Here's how the part is built. I have some questions about the finished solid (model axes, mm). Coordinates: 2 decimals unless noted, no trailing zeros. Loops run counter-clockwise (first coordinate to the right, second up) from the corner with the lowest first, then second, coordinate; pieces in that order, holes last. Notation, with made-up numbers: (36.25, 1) -> (47.25, 1) arc R27 cw to (47.25, 39) -> close; hole circle Ø11 at (-7.75, 75). An arc over 180 degrees is marked (long way). Answer as a JSON object with one key per item and string values. Group by question number.
1) I'm going to push a flat-ended pin straight in: pin 1 (1.9 mm diameter, centred on x = -181.44, z = -97.5, fed in from +Y). Where does the tip first touch, or does it pass through?
2) I need wall thicknesses on probe 1 along X at (y, z) = (1.35, -97.5); probe 2 along X at (y, z) = (1.5, -86); probe 3 along X at (y, z) = (1.6, -48). Which ranges of each line are inside material? Lowest first, please. Write a range as [from, to].
3) I want a section at A-A (z = -86). Write out the boundary of the cut face in (x, y), then the cut area to 3 significant figures.
4) I want a section at B-B (y = 0.65). Count the separate pieces of the cut face and the enclosed holes in it, then the cut area to 3 significant figures.
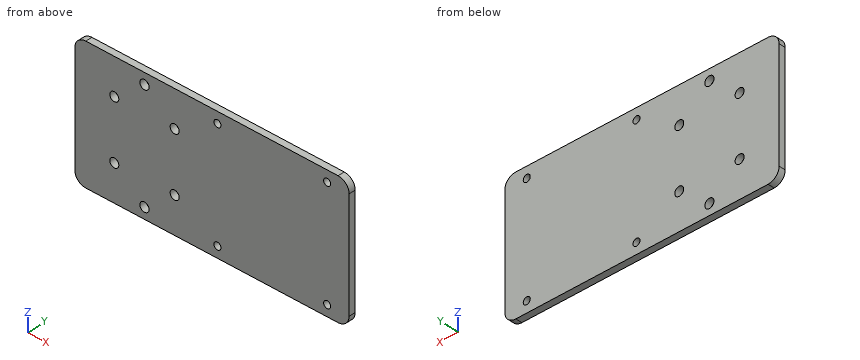
```python
from build123d import *

# Parameters (mm, degrees)
SKETCH_1_W          = 125
SKETCH_1_H          = 60
EXTRUDE_1_DEPTH     = 3
SKETCH_2_R          = 2.05
SKETCH_2_R_2        = 2.1
CUT_EXTRUDE_1_DEPTH = 267.924326413
SKETCH_3_R          = 1.6
CUT_EXTRUDE_2_DEPTH = 267.924326413
FILLET_1_R          = 5


with BuildPart() as part:
    # 草图1 → 凸台-拉伸1 (new body)
    with BuildSketch(Plane(origin=(0, 0, 0), x_dir=(1, 0, 0), z_dir=(0, 1, 0))):
        with Locations((-183.941364286, 72.5)):
            Rectangle(SKETCH_1_W, SKETCH_1_H)
    extrude(amount=EXTRUDE_1_DEPTH)

    # 草图2 → 切除-拉伸1 (cut, through all)
    with BuildSketch(Plane(origin=(0, 3, 0), x_dir=(1, 0, 0), z_dir=(0, 1, 0))):
        with Locations(Location((-228.441364286, 86, 0), (0, 0, 270))):
            Circle(SKETCH_2_R)
        with Locations(Location((-228.441364286, 59, 0), (0, 0, 270))):
            Circle(SKETCH_2_R)
        with Locations(Location((-200.941364286, 86, 0), (0, 0, 270))):
            Circle(SKETCH_2_R)
        with Locations(Location((-200.941364286, 59, 0), (0, 0, 90))):
            Circle(SKETCH_2_R)
        with Locations(Location((-214.691364286, 97.5, 0), (0, 0, 270))):
            Circle(SKETCH_2_R_2)
        with Locations(Location((-214.691364286, 47.5, 0), (0, 0, 90))):
            Circle(SKETCH_2_R_2)
    extrude(amount=-CUT_EXTRUDE_1_DEPTH, mode=Mode.SUBTRACT)

    # 草图3 → 切除-拉伸2 (cut, through all)
    with BuildSketch(Plane(origin=(0, 3, 0), x_dir=(1, 0, 0), z_dir=(0, 1, 0))):
        with Locations(Location((-181.441364286, 97.5, 0), (0, 0, 270))):
            Circle(SKETCH_3_R)
        with Locations(Location((-131.441364286, 97.5, 0), (0, 0, 270))):
            Circle(SKETCH_3_R)
        with Locations(Location((-131.441364286, 47.5, 0), (0, 0, 90))):
            Circle(SKETCH_3_R)
        with Locations(Location((-181.441364286, 47.5, 0), (0, 0, 90))):
            Circle(SKETCH_3_R)
    extrude(amount=-CUT_EXTRUDE_2_DEPTH, mode=Mode.SUBTRACT)

    # 圆角1
    fillet_1_edges = [part.edges().sort_by_distance(p)[0] for p in [
        (-121.441364286, 1.5, -42.5),
        (-246.441364286, 1.5, -42.5),
        (-246.441364286, 1.5, -102.5),
        (-121.441364286, 1.5, -102.5),
    ]]
    fillet(fillet_1_edges, radius=FILLET_1_R)


solid = part.part
```
Determined:
{
 "1": {"pin 1": "through"},
 "2": {"probe 1": "[-246.44, -216.79], [-212.59, -183.04], [-179.84, -133.04], [-129.84, -121.44]", "probe 2": "[-246.44, -230.49], [-226.39, -202.99], [-198.89, -121.44]", "probe 3": "[-246.44, -216.73], [-212.65, -182.96], [-179.92, -132.96], [-129.92, -121.44]"},
 "3": {"outline": "(-246.44, 0) -> (-230.49, 0) -> (-230.49, 3) -> (-246.44, 3) -> close; (-226.39, 0) -> (-202.99, 0) -> (-202.99, 3) -> (-226.39, 3) -> close; (-198.89, 0) -> (-121.44, 0) -> (-121.44, 3) -> (-198.89, 3) -> close", "area": "350 mm^2"},
 "4": {"separate pieces": "1", "enclosed holes": "10", "area": "7,370 mm^2"}
}
